Part model, mm, in its own coordinate system. Face numbers are marked on the shaded views. Coordinates: 2 decimals unless noted, no trailing zeros. Write each loop counter-clockwise with the first axis right and the second up, starting at its lowest first coordinate (ties: lowest second). Pieces come first, ordered by that corner, then holes. Notation, with made-up numbers: (58, 81.5) -> (85, 81.5) arc R17 cw to (85, 107.5) -> close; hole circle Ø8 at (63.5, 54). An arc over 180 degrees is marked (long way). Write item = value, one per line.
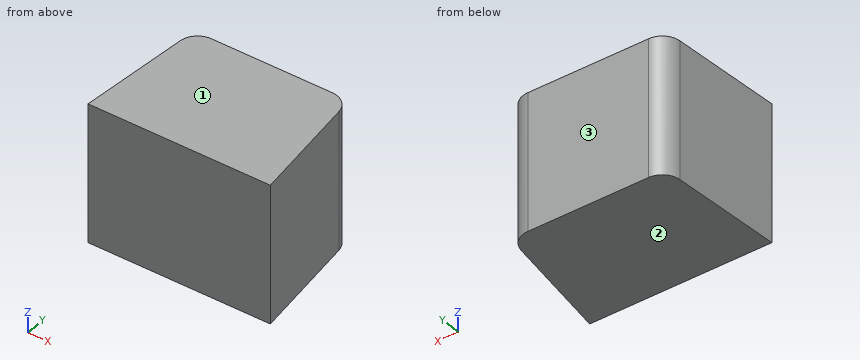
from build123d import *

# Parameters (mm, degrees)
BOSS_EXTRUDE3_DEPTH = 370
SKETCH3_W           = 569.98245323
SKETCH3_H           = 524.5
BOSS_EXTRUDE4_DEPTH = 100
BOSS_EXTRUDE5_DEPTH = 524.5
FILLET3_R           = 70


with BuildPart() as part:
    # Sketch1 → Boss-Extrude3 (new body)
    with BuildSketch(Plane(origin=(0, 0, 0), x_dir=(1, 0, 0), z_dir=(0, 1, 0))):
        Polygon((225.65, -262.25), (344.33245323, -262.25), (344.33245323, 262.25), (225.65, 262.25), (-225.65, 262.25), (-225.65, -262.25), align=None)
    extrude(amount=BOSS_EXTRUDE3_DEPTH)

    # Sketch3 → Boss-Extrude4 (add)
    with BuildSketch(Plane(origin=(0, 370, 0), x_dir=(1, 0, 0), z_dir=(0, 1, 0))):
        with Locations((59.341226615, 0)):
            Rectangle(SKETCH3_W, SKETCH3_H)
    extrude(amount=BOSS_EXTRUDE4_DEPTH)

    # Sketch6 → Boss-Extrude5 (add, through all)
    with BuildSketch(Plane.XY.offset(262.25)):
        Polygon((-225.65, 0), (-275.65, 0), (-225.65, 470), (344.33245323, 470), (394.33245323, 0), (344.33245323, 0), align=None)
    extrude(amount=-BOSS_EXTRUDE5_DEPTH)

    # Fillet3
    fillet3_edges = [part.edges().sort_by_distance(p)[0] for p in [
        (-225.65, 470, 0),
        (344.33245323, 470, 0),
    ]]
    fillet(fillet3_edges, radius=FILLET3_R)


solid = part.part
Q1. Pin check, flat tips, straight feed: pin 1 (1.5 mm diameter, centred on y = 409.5, z = 177, fed in from -X); pin 2 (12 mm diameter, centred on y = 253, z = -45.5, fed in from +X). Stop position of each tip, or through.
Model answer:
pin_1 = -232.15
pin_2 = 368.06
Q2. Probe line 1 (X direction, y = 382, z = -228); line 2 (Y direction, x = 292.5, z = -111.5); line 3 (X direction, y = 324, z = -77). List the from-to ranges inside material, lowest first. Write a range as from..to.
Model answer:
line_1 = -235.01..353.69
line_2 = 0..469.11
line_3 = -241.18..359.86
Q3. Saw through at C-C on y = 421. Give the cut face in (x, z), and give its area (3 significant figures).
Model answer:
outline = (-229.48, -262.25) -> (348.16, -262.25) -> (348.16, 262.25) -> (-229.48, 262.25) -> close
area = 303,000 mm²
Q4. Mould opens along Z. For the marked faces 1, 2 and 3 say: released by +Z, released by -Z, zero draft, split by the parting line, or undercut.
Model answer:
face_1 = released by +Z
face_2 = released by -Z
face_3 = zero draft
Q5. Saw through at A-A on z = -181.5. Give the cut face in (x, y).
Model answer:
outline = (-275.65, 0) -> (394.33, 0) -> (350.99, 407.41) arc R70 ccw to (281.38, 470) -> (-162.7, 470) arc R70 ccw to (-232.31, 407.41) -> close
Q6. Saw through at B-B on x = -220. Give the cut face in (y, z), and give its area (3 significant figures).
Model answer:
outline = (0, -262.25) -> (440.21, -262.25) -> (440.21, 262.25) -> (0, 262.25) -> close
area = 231,000 mm²
